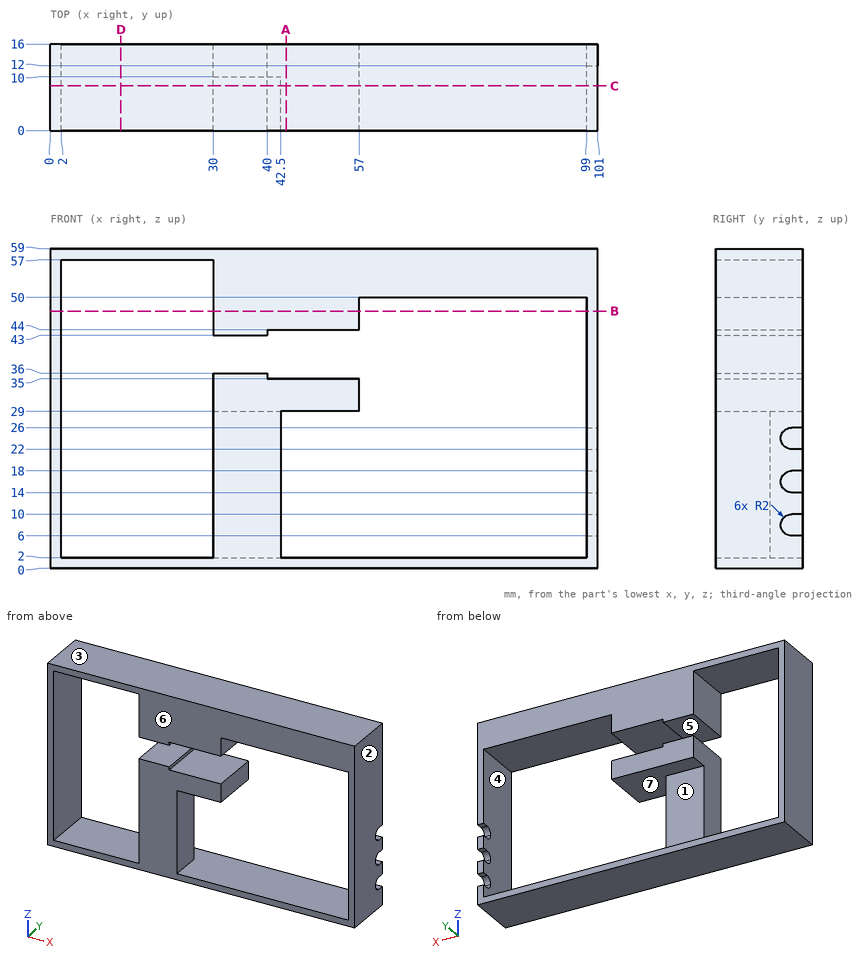
Design review of the part shown in the three views and the two pictorial views. Dimensions are in mm from the part's minimum x, y and z. A direction names the side the tool comes from. Round coordinates to 2 decimals unless told otherwise and drop trailing zeros. Order: outer loops, then holes, each group sorted by start corner. A loop starts at its lowest first (then second) coordinate and runs counter-clockwise, first axis right, second up. Notation, with made-up numbers: (34.5, 5.25) - (64.5, 5.25) arc R22 ccw to (64.5, 39.25) - close; hole circle Ø1 at (-3, 42). An arc over 180 degrees is marked (long way). One line per question, with ' | ' between items.
Item 1: Machinability: for the marked faces 5, 6 and 7, which of the approach directions +Z, -Z, +X, -X, +Y, -Y give a long, thin tool a straight path to every point of the face, cutting with its end or side? Answer none if there is none.
Checks:
face 5: +Y, -Y | face 6: +Z, -Z, +X, -X, -Y | face 7: +Y
Item 2: Take a section at D-D, the plane x = 13. Write out the cut boundary in (y, z).
Checks:
outline: (0, 0) - (16, 0) - (16, 2) - (0, 2) - close; (0, 57) - (16, 57) - (16, 59) - (0, 59) - close
Item 3: Draft analysis for pull direction Z (two halves, no side actions). For the marked faces 1, 2, 3 and 4, state which applies: +Z half, -Z half, draft (parallel to the pull), parting line (faces both ways), or undercut.
Checks:
face 1: undercut | face 2: draft | face 3: +Z half | face 4: undercut
Item 4: Wall thickness on line 1 (X direction, y = 1.75, z = 17); line 2 (Z direction, x = 53.5, y = 3.25); line 3 (X direction, y = 10, z = 30): over which ranges is each line inside the solid? List them lowest first. Write a range as [from, to].
Checks:
line 1: [0, 2], [30, 42.5], [99, 101] | line 2: [0, 2], [29, 35], [44, 59] | line 3: [0, 2], [30, 57], [99, 101]
Item 5: Take a section at B-B, the plane z = 47.5. Write out the cut boundary in (x, y).
Checks:
outline: (0, 0) - (2, 0) - (2, 16) - (0, 16) - close; (30, 0) - (57, 0) - (57, 16) - (30, 16) - close; (99, 0) - (101, 0) - (101, 16) - (99, 16) - close
Item 6: Take a section at A-A, the plane x = 43.5. Write out the cut boundary in (y, z).
Checks:
outline: (0, 0) - (16, 0) - (16, 2) - (0, 2) - close; (0, 29) - (16, 29) - (16, 35) - (0, 35) - close; (0, 44) - (16, 44) - (16, 59) - (0, 59) - close
Item 7: Take a section at C-C, the plane y = 8.25. Write out the cut boundary in (x, z), then the cut area to 3 significant figures.
Checks:
outline: (0, 0) - (101, 0) - (101, 59) - (0, 59) - close; hole (2, 2) - (30, 2) - (30, 36) - (40, 36) - (40, 35) - (57, 35) - (57, 29) - (42.5, 29) - (42.5, 2) - (99, 2) - (99, 50) - (57, 50) - (57, 44) - (40, 44) - (40, 43) - (30, 43) - (30, 57) - (2, 57) - close | area: 1,790 mm²
